The figure shows three views and two pictorial views of one solid part (mm, origin at its lowest corner). Answer the questions. A direction names the side the tool comes from. Give positions to 0.01 mm unless a question says otherwise; leave off trailing zeros. Loops run counter-clockwise (first coordinate to the right, second up) from the corner with the lowest first, then second, coordinate; pieces in that order, holes last. Notation, with made-up numbers: M -23.5,40 L 11.5,40 A18 cw 11.5,70 Z; hole C 75,38.5 d3. An arc over 180 degrees is marked long. One line per item, written item: value. Start each with the question number.
Q1. Flat-ended cylindrical pins translate along their axes: pin 1 (2 mm diameter, centred on x = 1.5, y = 2.5, fed in from -Z); pin 2 (1 mm diameter, centred on x = 11.5, y = 4.5, fed in from +Z). Find the tip coordinate at first contact, or state that the pin passes through.
Q2. The mould has two halves that part along Z. Classify the marked faces 1, 2 and 3: +Z half, -Z half, draft (parallel to the pull), parting line (faces both ways), or undercut.
Q3. For the marked faces 4, 5 and 6, determine the directions among +Z, -Z, +X, -X, +Y, -Y from which every point of the face is accessible in a straight line to the end or side of a thin tool.
Q4. Consider L1, parallel to Z at x = 6.75, y = 6.25 (1 decimal); L2, parallel to Y at x = 12.5, z = 4.5; L3, parallel to Z at x = 5.5, y = 6 (1 decimal). Determine where each line is inside the solid, lowest interval first.
Q5. A cutting plane is placed at C-C, the plane z = 10. Determine the outline of the cut face in (x, y) (1 decimal), and give its area (3 significant figures).
Q6. A cutting plane is placed at B-B, the plane x = 7. Determine the outline of the cut face in (y, z).
Q7. A cutting plane is placed at A-A, the plane y = 5.75. Determine the outline of the cut face in (x, z) (1 decimal).
Q8. A cutting plane is placed at D-D, the plane x = 2.75. Determine the outline of the cut face in (y, z).
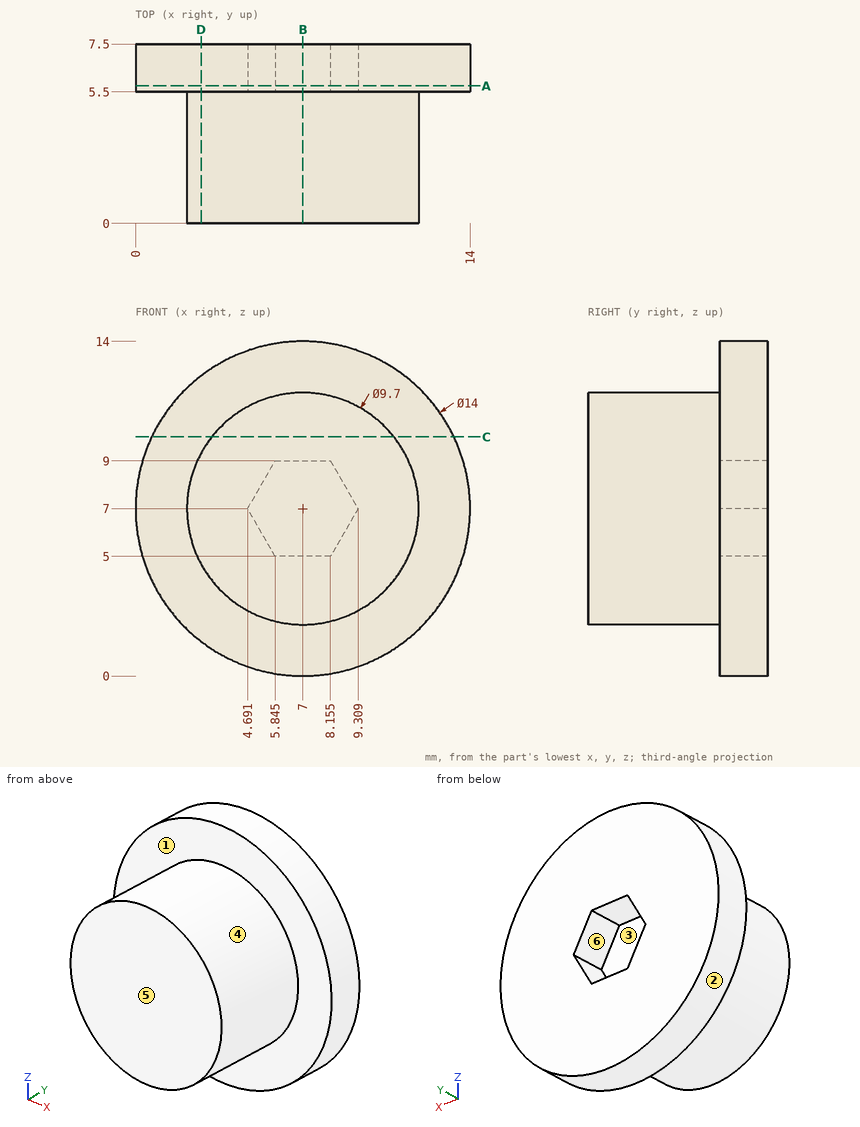
Answer block:
1. pin 1: z = 5.19
1. pin 2: z = 9.74
2. face 1: draft
2. face 2: parting line
2. face 3: undercut
3. face 4: -Y
3. face 5: +Z, -Z, +X, -X, -Y
3. face 6: +Y
4. L1: 0 to 5, 9 to 14
4. L2: 5.5 to 7.5
4. L3: 0.2 to 5.6, 8.4 to 13.8
5. outline: M 0.7,5.5 L 3.2,5.5 L 3.2,0 L 10.8,0 L 10.8,5.5 L 13.3,5.5 L 13.3,7.5 L 0.7,7.5 Z
5. area: 67.2 mm^2
6. outline: M 0,2.15 L 5.5,2.15 L 5.5,0 L 7.5,0 L 7.5,5 L 5.5,5 L 5.5,9 L 7.5,9 L 7.5,14 L 5.5,14 L 5.5,11.85 L 0,11.85 Z
7. outline: C 7,7 d14; hole M 4.7,7 L 5.8,5 L 8.2,5 L 9.3,7 L 8.2,9 L 5.8,9 Z
8. outline: M 0,4.66 L 5.5,4.66 L 5.5,1.44 L 7.5,1.44 L 7.5,12.56 L 5.5,12.56 L 5.5,9.34 L 0,9.34 Z
